from build123d import *

# Parameters (mm, degrees)
BOSS_EXTRUDE1_DEPTH    = 11
M5_CLEARANCE_HOLE1_D   = 5.5
CUT_EXTRUDE1_START     = -6
CUT_EXTRUDE1_OUTLINE_R = 2.75
CUT_EXTRUDE1_DEPTH     = 12
SKETCH1_4_R            = 3.25
CUT_EXTRUDE2_DEPTH     = 48.675989764
FILLET1_R              = 0.5


# Read off the part's stored shape, not the designer's step: Cut-Extrude1
with BuildPart() as part:
    # Sketch1 → Boss-Extrude1 (new, symmetric)
    with BuildSketch(Plane.XY):
        with BuildLine():
            Line((6, 0), (6, -40))
            ThreePointArc((6, -40), (0, -46), (-6, -40))
            Line((-6, -40), (-6, 0))
            ThreePointArc((-6, 0), (0, 6), (6, 0))
        make_face()
    extrude(amount=BOSS_EXTRUDE1_DEPTH, both=True)

    # M5 Clearance Hole1 (through all)
    with Locations(Plane.XY.offset(11)):
        with Locations((0, 0), (0, -15), (0, -30), (0, -40)):
            Hole(M5_CLEARANCE_HOLE1_D / 2)

    # Cut-Extrude1 outline → Cut-Extrude1 (cut)
    with BuildSketch(Plane.XY.offset(CUT_EXTRUDE1_START)):
        with BuildLine():
            Line((-6, -21), (0, -21))
            ThreePointArc((0, -21), (4.242640687, -19.242640687), (6, -15))
            Line((6, -15), (6, 0))
            ThreePointArc((6, 0), (0, 6), (-6, 0))
            Line((-6, 0), (-6, -21))
        make_face()
        with Locations((0, -15)):
            Circle(CUT_EXTRUDE1_OUTLINE_R, mode=Mode.SUBTRACT)
        Circle(CUT_EXTRUDE1_OUTLINE_R, mode=Mode.SUBTRACT)
    extrude(amount=CUT_EXTRUDE1_DEPTH, mode=Mode.SUBTRACT)

    # Sketch1_4 → Cut-Extrude2 (cut, through all)
    with BuildSketch(Plane.XY):
        Circle(SKETCH1_4_R)
        with Locations((0, -15)):
            Circle(SKETCH1_4_R)
    extrude(amount=-CUT_EXTRUDE2_DEPTH, mode=Mode.SUBTRACT)

    # Fillet1
    fillet1_edges = [part.edges().sort_by_distance(p)[0] for p in [
        (6, -15, 0),
    ]]
    fillet(fillet1_edges, radius=FILLET1_R)


solid = part.part
CAD build for the part. Positions are in the model's coordinates, mm. A direction names the side the tool comes from. Give positions to 0.01 mm unless a question says otherwise; leave off trailing zeros. Write each loop counter-clockwise with the first axis right and the second up, starting at its lowest first coordinate (ties: lowest second). Pieces come first, ordered by that corner, then holes. Notation, with made-up numbers: (72.25, 78) -> (116.25, 78) arc R11 cw to (116.25, 87) -> close; hole circle Ø10 at (30, -21.5). An arc over 180 degrees is marked (long way). Return JSON: item names as keys, results as strings.
Item 1: Band-saw the part on B-B (z = 5). List the corners of the cut face in (x, y).
Answer below:
{"outline": "(-6, -40) arc R6 ccw to (6, -40) -> (6, -18.46) arc R0.5 ccw to (5.08, -18.2) arc R6 cw to (0, -21) -> (-6, -21) -> close; hole circle Ø5.5 at (0, -40); hole circle Ø5.5 at (0, -30)"}
Item 2: Band-saw the part on A-A (y = -15). List the corners of the cut face in (x, z).
Answer below:
{"outline": "(-6, -11) -> (-3.25, -11) -> (-3.25, -6) -> (-6, -6) -> close; (-6, 6) -> (-2.75, 6) -> (-2.75, 11) -> (-6, 11) -> close; (2.75, 6) -> (6, 6) -> (6, 11) -> (2.75, 11) -> close; (3.25, -11) -> (6, -11) -> (6, -6) -> (3.25, -6) -> close"}
Item 3: Drill centre lines: probe 1 along Y at (x, z) = (0, 9.1); probe 2 along Y at (x, z) = (0, 5); probe 3 along Z at (x, y) = (-2.75, -11). Where is each one in solid material? Low to high.
Answer below:
{"probe 1": "y = -46 to -42.75, -37.25 to -32.75, -27.25 to -17.75, -12.25 to -2.75, 2.75 to 6", "probe 2": "y = -46 to -42.75, -37.25 to -32.75, -27.25 to -21", "probe 3": "z = -11 to -6, 6 to 11"}
Item 4: Drop flat-ended pins along their axis: pin 1 (5 mm diameter, centred on x = -4, z = -1, fed in from +Y); pin 2 (5 mm diameter, centred on x = 2, y = -2.5, fed in from -Z). Give the stop position or say it passes through.
Answer below:
{"pin 1": "stops at y = -21", "pin 2": "stops at z = -11"}
Item 5: Tool access for faces 4 (the flat face through (0, -7, -6)), 5 (the cylindrical face through (-0.423, -11.778, -8.465)), 6 (the cylindrical face through (5.647, -17.986, 0.084)): list every direction of +Z, -Z, +X, -X, +Y, -Y with a clear straight run to the whole face (end or side of a thin tool).
Answer below:
{"face 4": "-X, +Y", "face 5": "-Z", "face 6": "+Y"}
Item 6: Band-saw the part on C-C (x = -1.75). Give the number of separate pieces and of enclosed holes in the cut face, then the cut area to 3 significant figures.
Answer below:
{"separate pieces": "7", "enclosed holes": "0", "area": "528 mm2"}
Item 7: Two-plate mould, pull along Y, no slides. Class faces 1 (the flat face through (0, -20, 11)), 2 (the cylindrical face through (2.862, -20.273, -0.084)), 3 (the cylindrical face through (0.596, -2.685, 8.465)): +Y half, -Y half, draft (parallel to the pull), parting line (faces both ways), or undercut.
Answer below:
{"face 1": "draft", "face 2": "+Y half", "face 3": "undercut"}
Item 8: Band-saw the part on D-D (x = -4.75). List the corners of the cut face in (y, z).
Answer below:
{"outline": "(-43.67, -11) -> (3.67, -11) -> (3.67, -6) -> (-21, -6) -> (-21, 6) -> (3.67, 6) -> (3.67, 11) -> (-43.67, 11) -> close"}
